```python
from build123d import *

# Parameters (mm, degrees)
F0_R     = 1.5875
F1_DEPTH = 1.5748
F3_DEPTH = 3.175
F5_DEPTH = 3.175
F7_DEPTH = 4.7508
F9_DEPTH = 4.7508
F10_R    = 1.27
F11_SIZE = 1.27


with BuildPart() as f1:
    # F0 (on Front) → F1 (new body)
    with BuildSketch(Plane.XZ):
        with BuildLine():
            ThreePointArc((21.59, 10.16), (20.1021024484, 13.7521024484), (16.51, 15.24))
            Line((16.51, 15.24), (-16.51, 15.24))
            ThreePointArc((-16.51, 15.24), (-20.1021024484, 13.7521024484), (-21.59, 10.16))
            Line((-21.59, 10.16), (-21.59, -10.16))
            ThreePointArc((-21.59, -10.16), (-20.1021024484, -13.7521024484), (-16.51, -15.24))
            Line((-16.51, -15.24), (16.51, -15.24))
            ThreePointArc((16.51, -15.24), (20.1021024484, -13.7521024484), (21.59, -10.16))
            Line((21.59, -10.16), (21.59, 10.16))
        make_face()
        with Locations((-16.891, -10.414)):
            Circle(F0_R, mode=Mode.SUBTRACT)
        with Locations((16.891, -10.414)):
            Circle(F0_R, mode=Mode.SUBTRACT)
        with Locations((-16.891, 10.414)):
            Circle(F0_R, mode=Mode.SUBTRACT)
        with Locations((16.891, 10.414)):
            Circle(F0_R, mode=Mode.SUBTRACT)
    extrude(amount=F1_DEPTH)

    # F2 (on face) → F3 (join)
    with BuildSketch(Plane.XZ.offset(1.5748)):
        with BuildLine():
            ThreePointArc((-12.192, -3.048), (0, -15.24), (12.192, -3.048))
            ThreePointArc((12.192, -3.048), (0, 9.144), (-12.192, -3.048))
        make_face()
        with BuildLine():
            ThreePointArc((-12.192, -3.048), (0, 9.144), (12.192, -3.048))
            Line((12.192, -3.048), (12.192, 15.24))
            Line((12.192, 15.24), (-12.192, 15.24))
            Line((-12.192, 15.24), (-12.192, -3.048))
        make_face()
    extrude(amount=F3_DEPTH)

    # F4 (on Front) → F5 (cut)
    with BuildSketch(Plane.XZ):
        with BuildLine():
            ThreePointArc((-10.668, -3.048), (0, -13.716), (10.668, -3.048))
            ThreePointArc((10.668, -3.048), (0, 7.62), (-10.668, -3.048))
        make_face()
        with BuildLine():
            ThreePointArc((-10.668, -3.048), (0, 7.62), (10.668, -3.048))
            Line((10.668, -3.048), (10.668, 15.24))
            Line((10.668, 15.24), (-10.668, 15.24))
            Line((-10.668, 15.24), (-10.668, -3.048))
        make_face()
    extrude(amount=F5_DEPTH, mode=Mode.SUBTRACT)

    # F6 (on face) → F7 (cut, through all)
    with BuildSketch(Plane.XZ.offset(4.7498)):
        with BuildLine():
            Line((5.715, -3.048), (5.715, 15.24))
            Line((5.715, 15.24), (-5.715, 15.24))
            Line((-5.715, 15.24), (-5.715, -3.048))
            ThreePointArc((-5.715, -3.048), (0, 2.667), (5.715, -3.048))
        make_face()
        with BuildLine():
            ThreePointArc((-5.715, -3.048), (0, -8.763), (5.715, -3.048))
            ThreePointArc((5.715, -3.048), (0, 2.667), (-5.715, -3.048))
        make_face()
    extrude(amount=-F7_DEPTH, mode=Mode.SUBTRACT)

    # F8 (on face) → F9 (cut, through all)
    with BuildSketch(Plane.XZ.offset(4.7498)):
        with BuildLine():
            Line((-5.715, 15.24), (-8.255, 15.24))
            ThreePointArc((-8.255, 15.24), (-6.4589487758, 14.4960512242), (-5.715, 12.7))
            Line((-5.715, 12.7), (-5.715, 15.24))
        make_face()
        with BuildLine():
            Line((5.715, 15.24), (5.715, 12.7))
            ThreePointArc((5.715, 12.7), (6.4589487758, 14.4960512242), (8.255, 15.24))
            Line((8.255, 15.24), (5.715, 15.24))
        make_face()
    extrude(amount=-F9_DEPTH, mode=Mode.SUBTRACT)

    # F10
    f10_edges = [f1.edges().sort_by_distance(p)[0] for p in [
        (0, -4.7498, -15.24),
        (-12.192, -4.7498, 6.096),
        (12.192, -4.7498, 6.096),
    ]]
    fillet(f10_edges, radius=F10_R)

    # F11
    f11_edges = [f1.edges().sort_by_distance(p)[0] for p in [
        (-18.4785, -1.5748, 10.414),
        (-18.4785, -1.5748, -10.414),
        (15.3035, -1.5748, 10.414),
        (15.3035, -1.5748, -10.414),
    ]]
    chamfer(f11_edges, length=F11_SIZE)


solid = f1.part
```
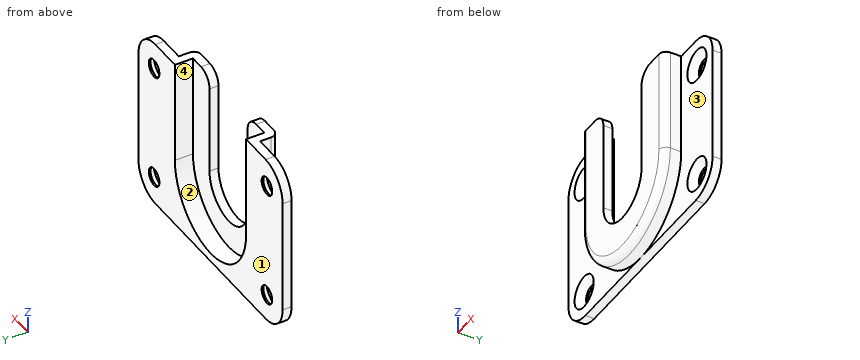
Verification items for the finished model (mm, model axes). Face numbers are marked on the shaded views. A direction names the side the tool comes from. Coordinates: 2 decimals unless noted, no trailing zeros. Write each loop counter-clockwise with the first axis right and the second up, starting at its lowest first coordinate (ties: lowest second). Pieces come first, ordered by that corner, then holes. Notation, with made-up numbers: M 33,49.25 L 69,49.25 A14 ccw 69,67.25 Z; hole C 60.5,50.25 d2. An arc over 180 degrees is marked long. Answer as a JSON object with one key per item and string values. Group by question number.
(1) Cross-section at C-C, the plane z = -11. State how many separate pieces and enclosed holes the cut face has, and give its area (3 significant figures).
(2) Gauge pin test, flat ends, axial feed: pin 1 (10.5 mm diameter, centred on x = -1, z = -5.5, fed in from +Y) (3 decimals); pin 2 (1.5 mm diameter, centred on y = -2, z = 5, fed in from -X); pin 3 (0.6 mm diameter, centred on y = -3, z = 7, fed in from +X); pin 4 (1.7 mm diameter, centred on y = -3.5, z = 1, fed in from -X). Record the tip position at first contact, or that the pin passes through.
(3) Cross-section at B-B, the plane y = -2.45. Record the cut outline in (x, z).
(4) Tool access check on the marked faces 1 and 2. Record the directions out of +Z, -Z, +X, -X, +Y, -Y that give a thin tool (end or side, any length) a straight path to the whole face; none if there is none.
(5) Material ranges on line 1 (X direction, y = -1.75, z = 4.5); line 2 (Y direction, x = 7.5, z = -6) (3 decimals); line 3 (X direction, y = -0.9, z = 5.5), recorded low to high.
(6) Release check for a two-part mould opening along X. For the marked faces 3 and 4 record: +X half, -X half, draft (parallel to the pull), parting line (faces both ways), or undercut.
(7) Cross-section at A-A, the plane z = 7. Record the cut outline in (x, y) (3 decimals), and give its area (3 significant figures).
Reply:
{
 "1": {"separate pieces": "3", "enclosed holes": "0", "area": "67.7 mm²"},
 "2": {"pin 1": "y = -3.175", "pin 2": "x = -21.59", "pin 3": "x = 12.19", "pin 4": "x = -12.19"},
 "3": {"outline": "M -12.19,-3.05 A12.19 ccw 12.19,-3.05 L 12.19,15.24 L 10.67,15.24 L 10.67,-3.05 A10.67 cw -10.67,-3.05 L -10.67,15.24 L -12.19,15.24 Z"},
 "4": {"face 1": "+Z, -Z, +X, -X, +Y", "face 2": "+Z, +Y"},
 "5": {"line 1": "-12.19 to -10.67, 10.67 to 12.19", "line 2": "-4.75 to -3.175", "line 3": "-21.59 to -10.67, 10.67 to 21.59"},
 "6": {"face 3": "draft", "face 4": "undercut"},
 "7": {"outline": "M -21.59,-1.575 L -12.192,-1.575 L -12.192,-3.48 A1.27 ccw -10.922,-4.75 L -5.715,-4.75 L -5.715,-3.175 L -10.668,-3.175 L -10.668,0 L -21.59,0 Z; M 5.715,-4.75 L 10.922,-4.75 A1.27 ccw 12.192,-3.48 L 12.192,-1.575 L 21.59,-1.575 L 21.59,0 L 10.668,0 L 10.668,-3.175 L 5.715,-3.175 Z", "area": "59.0 mm²"}
}
